Part model, mm, in its own coordinate system. A direction names the side the tool comes from. Give positions to 0.01 mm unless a question says otherwise; leave off trailing zeros. Write each loop counter-clockwise with the first axis right and the second up, starting at its lowest first coordinate (ties: lowest second). Pieces come first, ordered by that corner, then holes. Notation, with made-up numbers: M 47.5,55.25 L 68.5,55.25 A12 cw 68.5,63.25 Z; hole C -10.5,66 d4. An arc over 180 degrees is marked long. Use CSV: the item, a comma, the result in double quotes. Start each with the question number.
Item 1: Pin check, flat tips, straight feed: pin 1 (12 mm diameter, centred on x = 6.5, z = -10.5, fed in from +Y); pin 2 (2 mm diameter, centred on x = 3.5, z = 10, fed in from +Y); pin 3 (10 mm diameter, centred on y = 13.5, z = 3.5, fed in from +X). Stop position of each tip, or through.
Item 2: Cut at C-C (z = -8). List the corners of the cut face in (x, y).
Item 3: Drill centre lines: line 1 (Z direction, x = -18, y = 11.5); line 2 (Y direction, x = 0, z = -2.25); line 3 (X direction, y = 3.5, z = 5.25). Where is each one in solid material? Low to high. Write a range as [from, to].
Item 4: Mould opens along Y. For faces 3 (the cylindrical face through (12.774, 20.035, 14.747)), 4 (the cylindrical face through (2.676, 4.198, 0.21)), 5 (the flat face through (0, 6, 15)) say: released by +Y, released by -Y, zero draft, split by the parting line, or undercut.
Item 5: Which spindle directions (+Z, -Z, +X, -X, +Y, -Y) get a long thin tool onto all of the face, cutting with end or side? Do faces 1 (the flat face through (10, -18, 12.5)), 2 (the cylindrical face through (12.774, 20.035, -14.747)). Say none if no direction does.
Item 6: Cut at A-A (y = 0). List the corners of the cut face in (x, z), then the cut area to 3 significant figures.
from build123d import *

# Parameters (mm, degrees)
CROQUIS1_R                 = 20
SALIENTE_EXTRUIR1_DEPTH    = 12.5
CROQUIS2_R                 = 23.760562535
SALIENTE_EXTRUIR2_DEPTH    = 2.5
CHAFL_N1_SIZE              = 2
CHAFL_N1_OF_SIMETR_A1_SIZE = 2
CROQUIS3_R                 = 4.978571234
CORTAR_EXTRUIR1_DEPTH      = 46.045850685


with BuildPart() as part:
    # Croquis1 → Saliente-Extruir1 (new, symmetric)
    with BuildSketch(Plane.XY):
        Circle(CROQUIS1_R)
    extrude(amount=SALIENTE_EXTRUIR1_DEPTH, both=True)

    # Croquis2 → Saliente-Extruir2 (add)
    with BuildSketch(Plane.XY.offset(12.5)):
        Circle(CROQUIS2_R)
    saliente_extruir2 = extrude(amount=SALIENTE_EXTRUIR2_DEPTH)

    # Chaflán1
    chafl_n1_edges = [part.edges().sort_by_distance(p)[0] for p in [
        (-23.760562535, 0, 12.5),
    ]]
    chamfer(chafl_n1_edges, length=CHAFL_N1_SIZE)

    # Simetría1: Saliente-Extruir2 across plane
    add(saliente_extruir2.mirror(Plane.XY))

    # Chaflán1 of Simetría1
    chafl_n1_of_simetr_a1_edges = [part.edges().sort_by_distance(p)[0] for p in [
        (-23.760562535, 0, -12.5),
    ]]
    chamfer(chafl_n1_of_simetr_a1_edges, length=CHAFL_N1_OF_SIMETR_A1_SIZE)

    # Croquis3 → Cortar-Extruir1 (cut, through all)
    with BuildSketch(Plane.XY.offset(15)):
        Circle(CROQUIS3_R)
    extrude(amount=-CORTAR_EXTRUIR1_DEPTH, mode=Mode.SUBTRACT)


solid = part.part
Worked answers:
1,pin 1,"stops at y = 23.67"
1,pin 2,"stops at y = 19.84"
1,pin 3,"stops at x = 18.1"
2,outline,"C 0,0 d40; hole C 0,0 d9.96"
3,line 1,"z = [-15, -12.5], [12.5, 15]"
3,line 2,"y = [-20, -4.98], [4.98, 20]"
3,line 3,"x = [-19.69, -3.54], [3.54, 19.69]"
4,face 3,"split by the parting line"
4,face 4,"undercut"
4,face 5,"zero draft"
5,face 1,"none"
5,face 2,"+Z, -Z"
6,outline,"M -23.76,-15 L -4.98,-15 L -4.98,15 L -23.76,15 L -23.76,14.5 L -21.76,12.5 L -20,12.5 L -20,-12.5 L -21.76,-12.5 L -23.76,-14.5 Z; M 4.98,-15 L 23.76,-15 L 23.76,-14.5 L 21.76,-12.5 L 20,-12.5 L 20,12.5 L 21.76,12.5 L 23.76,14.5 L 23.76,15 L 4.98,15 Z"
6,area,"931 mm^2"
